The listing builds one solid part. Answer for the finished solid, in the listing's coordinates (mm). A direction names the side the tool comes from. Coordinates: 2 decimals unless noted, no trailing zeros. Write each loop counter-clockwise with the first axis right and the second up, starting at its lowest first coordinate (ties: lowest second). Pieces come first, ordered by that corner, then holes.
Autodesk Inventor part; units mm, degrees
ref_plane "YZ Plane" through (0, 0, 0) normal (1, 0, 0) x (0, 1, 0)
ref_plane "XZ Plane" through (0, 0, 0) normal (0, 1, 0) x (-1, 0, 0)
ref_plane "XY Plane" through (0, 0, 0) normal (0, 0, 1) x (1, 0, 0)
sketch "Sketch1" plane through (0, 0, 0) normal (0, 0, 1) x (1, 0, 0)
  line L0 (-31.75, 5.08) -> (31.75, 5.08)
  line L1 (31.75, 5.08) -> (31.75, -5.08)
  line L2 (31.75, -5.08) -> (-31.75, -5.08)
  line L3 (-31.75, -5.08) -> (-31.75, 5.08)
  point P0 (0, 0)
  dimension "d0" = 63.5
  dimension "d3" = 31.75
  dimension "d4" = 10.16
  dimension "d17" = 5.08
extrude "Extrusion1" add sketch "Sketch1" along normal blind 76.2
sketch "Sketch3" plane through (0, 0, 76.2) normal (0, 0, 1) x (1, 0, 0)
  line L0 (-27.25, 0.3875) -> (27.25, 0.3875)
  line L1 (27.25, 0.3875) -> (27.25, -0.3745)
  line L2 (27.25, -0.3745) -> (-27.25, -0.3745)
  line L3 (-27.25, -0.3745) -> (-27.25, 0.3875)
  line L4 (-31.75, 5.08) -> (-31.75, -5.08)
  point P0 (0, 0)
  point P1 (-27.25, 0.0065)
  dimension "d6" = 0.762
  dimension "d7" = 54.5
  dimension "d8" = 4.5
extrude "Extrusion2" cut sketch "Sketch3" against normal blind 85.1
sketch "Sketch8" plane through (0, 0, 76.2) normal (0, 0, 1) x (1, 0, 0)
  line L0 (-31.75, -5.08) -> (31.75, -5.08)
  line L1 (31.75, -5.08) -> (31.75, 5.08)
  line L2 (-31.75, -5.08) -> (31.75, -5.08)
  line L3 (31.75, -5.08) -> (31.75, 0.3875)
  line L4 (31.75, 0.3875) -> (-31.75, 0.3875)
  line L5 (27.25, 0.3875) -> (27.25, -0.3745)
  line L6 (27.25, -0.3745) -> (-27.25, -0.3745)
  line L7 (-27.25, -0.3745) -> (-27.25, 0.3875)
  line L8 (-27.25, 0.3875) -> (27.25, 0.3875)
  line L9 (-31.75, -5.08) -> (31.75, -5.08)
  line L10 (31.75, -5.08) -> (31.75, 5.08)
  line L11 (31.75, 5.08) -> (-31.75, 5.08)
  line L12 (-31.75, 5.08) -> (-31.75, -5.08)
  line L13 (-27.25, 0.3875) -> (-27.25, -0.3745)
  line L14 (-27.25, 0.3875) -> (27.25, 0.3875)
  line L15 (27.25, 0.3875) -> (27.25, -5.08)
  line L16 (27.25, -5.08) -> (-27.25, -5.08)
  line L17 (-27.25, -5.08) -> (-27.25, 0.3875)
  point P0 (0, 0)
  dimension "d30" = 0
sketch "Sketch9" plane through (-31.75, 5.08, 0) normal (0, 1, 0) x (1, 0, 0)
  line L0 (28.35, -18.7333) -> (35.15, -18.7333)
  line L1 (35.15, -18.7333) -> (35.15, -39.7333)
  line L2 (35.15, -39.7333) -> (28.35, -39.7333)
  line L3 (28.35, -39.7333) -> (28.35, -18.7333)
  line L4 (0, 0) -> (0, -76.2)
  line L5 (63.5, 0) -> (0, 0)
  point P0 (31.75, 0)
  point P1 (0, -38.1)
  dimension "d31" = 21
  dimension "d32" = 6.8
  dimension "d33" = 28.35
  dimension "d34" = 18.7333
extrude "Extrusion6" cut sketch "Sketch8" against normal blind 76.2 contours L17 L6 L15 L0
sketch "Sketch11" plane through (0, 0, 76.2) normal (0, 0, 1) x (1, 0, 0)
  point P0 (0, 0)
sketch "Sketch12" plane through (-31.75, -5.08, 0) normal (0, -1, 0) x (1, 0, 0)
  line L0 (4.5, 0) -> (4.5, 76.2)
  line L1 (0, 76.2) -> (4.5, 76.2)
  line L2 (0, 0) -> (0, 76.2)
  line L3 (0, 0) -> (4.5, 0)
  line L4 (59, 76.2) -> (59, 0)
  line L5 (59, 0) -> (63.5, 0)
  line L6 (63.5, 0) -> (63.5, 76.2)
  line L7 (59, 76.2) -> (63.5, 76.2)
  point P0 (31.75, 0)
extrude "Extrusion7" add sketch "Sketch12" along normal blind 3.641
sketch "Sketch14" plane through (27.25, 0.3875, 0) normal (-1, 0, 0) x (0, 0, 1)
  circle A0 centre (10.16, -3.3935) radius 2.55
  line L0 (76.2, 0) -> (0, 0)
  line L1 (76.2, -9.1085) -> (0, -9.1085)
  line L2 (0, -9.1085) -> (0, 0)
  point P0 (0, -0.3875)
  dimension "d41" = 5.1
  dimension "d43" = 5.715
  dimension "d44" = 10.16
extrude "Extrusion9" cut sketch "Sketch14" against normal blind 25.4
sketch "Sketch17" plane through (-31.75, -8.721, 0) normal (0, -1, 0) x (1, 0, 0)
  circle A0 centre (61.25, 3.81) radius 1.05
  line L0 (59, 0) -> (63.5, 0)
  line L1 (59, 76.2) -> (59, 0)
  circle A1 centre (2.25, 3.81) radius 1.05
  line L2 (0, 76.2) -> (0, 0)
  line L3 (0, 0) -> (4.5, 0)
  circle A2 centre (2.25, 72.39) radius 1.05
  circle A3 centre (61.25, 72.39) radius 1.05
  line L4 (4.5, 76.2) -> (0, 76.2)
  line L5 (63.5, 76.2) -> (59, 76.2)
  point P0 (31.75, 0)
  dimension "d98" = 2.1
  dimension "d99" = 3.81
  dimension "d100" = 2.25
  dimension "d101" = 2.25
  dimension "d102" = 2.1
  dimension "d103" = 3.81
  dimension "d104" = 2.1
  dimension "d105" = 2.1
  dimension "d106" = 3.81
  dimension "d107" = 3.81
  dimension "d108" = 2.25
extrude "Extrusion11" cut sketch "Sketch17" against normal blind 5.08
sketch "Sketch18" plane through (-27.25, 0.3875, 76.2) normal (0, -1, 0) x (1, 0, 0)
  circle A0 centre (5.5, -23.82) radius 1.25
  circle A1 centre (5.5, -12.42) radius 1.05
  circle A2 centre (5.5, -12.42) radius 1.25
  line L0 (3.5, -28.62) -> (3.5, -7.62)
  circle A3 centre (5.5, -23.82) radius 1.05
  line L1 (54.5, -28.62) -> (3.5, -28.62)
  line L2 (3.5, -7.62) -> (54.5, -7.62)
  circle A4 centre (52.5, -12.42) radius 1.05
  circle A5 centre (52.5, -12.42) radius 1.25
  line L3 (54.5, -7.62) -> (54.5, -28.62)
  circle A6 centre (52.5, -23.82) radius 1.05
  circle A7 centre (52.5, -23.82) radius 1.25
  line L4 (0, 0) -> (54.5, 0)
  line L5 (54.5, 0) -> (54.5, -76.2)
  point P0 (27.25, -76.2)
  dimension "d111" = 21
  dimension "d112" = 51
  dimension "d113" = 2.1
  dimension "d114" = 2.1
  dimension "d115" = 2.1
  dimension "d116" = 2.1
  dimension "d117" = 2
  dimension "d118" = 2
  dimension "d119" = 2
  dimension "d120" = 2
  dimension "d121" = 11.4
  dimension "d122" = 4.8
  dimension "d123" = 11.4
  dimension "d124" = 4.8
  dimension "d125" = 0.2
  dimension "d126" = 0.2
  dimension "d127" = 0.2
  dimension "d128" = 0.2
  dimension "d131" = 7.62
  dimension "d132" = 0
extrude "Extrusion12" cut sketch "Sketch18" against normal blind 25.4 contours A0 | A1 | A2 | A3 | A4 | A5 | A6 | A7
sketch "Sketch21" plane through (-31.75, -8.721, 0) normal (0, -1, 0) x (1, 0, 0)
  line L0 (59, 76.2) -> (59, 0)
  line L1 (59, 69.5452) -> (61.2521, 69.5452)
  line L2 (61.2521, 69.5452) -> (61.2521, 46.6852)
  line L3 (61.2521, 46.6852) -> (59, 46.6852)
  line L4 (59, 46.6852) -> (59, 69.5452)
  line L5 (63.5, 0) -> (63.5, 76.2)
  line L6 (63.5, 76.2) -> (59, 76.2)
  point P0 (31.75, 0)
  dimension "d147" = 4.5
  dimension "d148" = 2.2479
  dimension "d149" = 6.6548
  dimension "d150" = 22.86
sketch "Sketch22" plane through (31.75, 5.08, 76.2) normal (1, 0, 0) x (0, 0, -1)
  line L0 (13.67, -4.6925) -> (13.67, 0)
  line L1 (13.67, -4.6925) -> (13.67, 0)
  line L2 (25.07, -4.6925) -> (25.07, 0)
  line L3 (22.57, -4.6925) -> (22.57, 0)
  line L4 (11.17, -4.6925) -> (11.17, 0)
  line L5 (23.8, -2.1525) -> (12.44, -2.1525)
  line L6 (12.44, -2.1525) -> (12.44, -11.0425)
  line L7 (12.44, -11.0425) -> (23.8, -11.0425)
  line L8 (23.8, -11.0425) -> (23.8, -2.1525)
  point P0 (76.2, -5.08)
  point P1 (24.97, -4.6925)
  point P2 (24.97, -2.1525)
  point P3 (11.27, -2.6605)
  point P4 (11.27, -4.6925)
  dimension "d152" = 8.89
  dimension "d153" = 2.54
  dimension "d169" = 1.27
  dimension "d170" = 1.27
extrude "Extrusion15" cut sketch "Sketch22" against normal blind 4.5212
sketch "Sketch24" plane through (31.75, 5.08, 76.2) normal (1, 0, 0) x (0, 0, -1)
  line L0 (38.6849, -4.6925) -> (33.6849, -4.6925)
  line L1 (33.6849, -4.6925) -> (33.6849, -8.6925)
  line L2 (33.6849, -8.6925) -> (38.6849, -8.6925)
  line L3 (38.6849, -8.6925) -> (38.6849, -4.6925)
  line L4 (0, -4.6925) -> (76.2, -4.6925)
  point P0 (76.2, -5.08)
  point P1 (23.8, -4.6925)
  dimension "d163" = 5
  dimension "d164" = 4
  dimension "d165" = 0
extrude "Extrusion16" cut sketch "Sketch24" against normal blind 9.1211
sketch "Sketch27" plane through (-27.25, 0.3875, 76.2) normal (0, -1, 0) x (1, 0, 0)
  line L0 (54.5, 0) -> (54.5, -76.2)
  line L1 (0, 0) -> (0, -76.2)
  line L2 (54.5, -29.89) -> (0, -29.89)
  line L3 (0, -29.89) -> (0, -6.35)
  line L4 (0, -6.35) -> (54.5, -6.35)
  line L5 (54.5, -6.35) -> (54.5, -29.89)
  line L6 (54.5, -28.62) -> (3.5, -28.62)
  line L7 (3.5, -7.62) -> (54.5, -7.62)
  point P0 (27.25, -76.2)
  point P1 (54.5, -6.35)
  point P2 (0, -29.89)
  dimension "d171" = 1.27
  dimension "d172" = 1.27
extrude "Extrusion17" cut sketch "Sketch27" against normal blind 1.5
sketch "Sketch30" plane through (-27.25, 0.3875, 0) normal (0, -1, 0) x (1, 0, 0)
  line L0 (39.9458, 42.5) -> (14.5458, 42.5)
  line L1 (14.5458, 42.5) -> (14.5458, 10.75)
  line L2 (14.5458, 10.75) -> (39.9458, 10.75)
  line L3 (39.9458, 10.75) -> (39.9458, 42.5)
  line L4 (23.85, 39.7333) -> (30.65, 39.7333)
  line L5 (54.5, 0) -> (0, 0)
  line L6 (54.5, 76.2) -> (54.5, 0)
  line L7 (0, 0) -> (0, 76.2)
  line L8 (36.9458, 38) -> (17.5458, 38)
  line L9 (17.5458, 38) -> (17.5458, 15.25)
  line L10 (17.5458, 15.25) -> (36.9458, 15.25)
  line L11 (36.9458, 15.25) -> (36.9458, 38)
  circle A0 centre (37.9458, 40.5) radius 1.25
  line L12 (54.5, 46.31) -> (0, 46.31)
  circle A1 centre (37.9458, 12.75) radius 1.25
  circle A2 centre (16.5458, 12.75) radius 1.25
  circle A3 centre (16.5458, 40.5) radius 1.25
  line L13 (54.5, 46.31) -> (0, 46.31)
  line L14 (0, 46.31) -> (0, 0)
  line L15 (54.5, 0) -> (0, 0)
  line L16 (54.5, 37.5151) -> (54.5, 0)
  line L17 (59, 37.5151) -> (54.5, 37.5151)
  line L18 (59, 42.5151) -> (59, 37.5151)
  line L19 (59, 42.5151) -> (54.5, 42.5151)
  line L20 (54.5, 46.31) -> (54.5, 42.5151)
  line L21 (41.8508, 44.405) -> (12.6408, 44.405)
  line L22 (12.6408, 44.405) -> (12.6408, 8.845)
  line L23 (12.6408, 8.845) -> (41.8508, 8.845)
  line L24 (41.8508, 8.845) -> (41.8508, 44.405)
  point P0 (27.25, 0)
  dimension "d177" = 31.75
  dimension "d178" = 25.4
  dimension "d179" = 54.5
  dimension "d180" = 14.5542
  dimension "d181" = 4.5
  dimension "d182" = 3.81
  dimension "d183" = 3
  dimension "d184" = 4.5
  dimension "d185" = 3
  dimension "d186" = 2.5
  dimension "d187" = 2
  dimension "d188" = 2
  dimension "d189" = 2.5
  dimension "d190" = 2.5
  dimension "d191" = 2.5
  dimension "d193" = 2
  dimension "d195" = 2
  dimension "d196" = 2
  dimension "d197" = 2
  dimension "d204" = 1.905
  dimension "d210" = 2
  dimension "d211" = 2
extrude "Extrusion18" cut sketch "Sketch30" against normal blind 25.4 contours L11 L10 L9 L8
extrude "Extrusion19" cut sketch "Sketch30" against normal blind 1.5 contours L3 L2 L1 L0 | L11 L10 L9 L8 | A0 | A1 | A2 | A3 | L24 L23 L22 L21
extrude "Extrusion20" cut sketch "Sketch30" against normal blind 254 contours A0 | A1 | A2 | A3
properties part number "Scanner_Test_Top"
1. Find the intervals of material crossed by L1, parallel to Z at x = -29.5, y = -6.8; L2, parallel to X at y = -6, z = 34.5; L3, parallel to Z at x = -5.5, y = 3, in increasing order.
Results found:
L1: z = 0 to 2.76, 4.86 to 71.34, 73.44 to 76.2
L2: x = -31.75 to -27.25, 27.25 to 31.75
L3: z = 0 to 15.25, 38 to 76.2
2. Section A-A on x = 25.25 is taken. Give the vertices of the cut face in (y, z).
Results found:
outline: (0.39, 0) - (5.08, 0) - (5.08, 51.13) - (1.89, 51.13) - (1.89, 46.31) - (0.39, 46.31) - close; (0.39, 69.85) - (1.89, 69.85) - (1.89, 65.03) - (5.08, 65.03) - (5.08, 76.2) - (0.39, 76.2) - close; (1.89, 53.63) - (5.08, 53.63) - (5.08, 62.53) - (1.89, 62.53) - close
3. Flat-ended cylindrical pins translate along their axes: P1, Ø4, axis at x = -21.75, z = 63.78, coming from the -Y side; P2, Ø8, axis at x = -15, z = 12, coming from the -Y side; P3, Ø0.6, axis at x = -29.5, z = 73, coming from the -Y side; P4, Ø2, axis at x = 25.25, z = 52.38, coming from the -Y side. Find the tip coordinate at first contact, or state that the pin passes through.
Results found:
P1: stops at y = 1.89
P2: stops at y = 0.39
P3: stops at y = -3.64
P4: passes through
4. Section D-D on y = -1.5 is taken. Give the vertices of the cut face in (x, z).
Results found:
outline: (-31.75, 0) - (-27.25, 0) - (-27.25, 76.2) - (-31.75, 76.2) - close; (27.25, 0) - (31.75, 0) - (31.75, 8.1) - (27.25, 8.1) - close; (27.25, 12.22) - (31.75, 12.22) - (31.75, 37.52) - (27.25, 37.52) - close; (27.25, 42.52) - (31.75, 42.52) - (31.75, 52.4) - (27.25, 52.4) - close; (27.25, 63.76) - (31.75, 63.76) - (31.75, 76.2) - (27.25, 76.2) - close
5. A tool of negligible diameter and unlimited length cuts with its end or side. For faces 5 (the flat face through (0, 0.388, 73)), 6 (the flat face through (0, 3, 15.25)), 7 (the flat face through (31.75, -5, 38)), 8 (the cylindrical face through (30.5, -6.22, 4.13)), 9 (the flat face through (30, -5.962, 58)), from which of +Z, -Z, +X, -X, +Y, -Y can it reach the whole face along a straight path? Write none if from no direction.
Results found:
face 5: +Z, -Z, -Y
face 6: +Y, -Y
face 7: +Z, -Z, +X, +Y, -Y
face 8: -Y
face 9: +X
6. Section B-B on z = 10.16 is taken. Give the vertices of the cut face in (x, y), then the cut area to 3 significant figures.
Results found:
outline: (-31.75, -8.72) - (-27.25, -8.72) - (-27.25, 0.39) - (-14.61, 0.39) - (-14.61, 1.89) - (14.6, 1.89) - (14.6, 0.39) - (27.25, 0.39) - (27.25, -0.46) - (31.75, -0.46) - (31.75, 5.08) - (-31.75, 5.08) - close; (27.25, -8.72) - (31.75, -8.72) - (31.75, -5.56) - (27.25, -5.56) - close
area: 313 mm2
7. For a pull along Z with two mould halves and no side action, classify faces 1 (the flat face through (0, 5.08, 46)), 2 (the flat face through (0, 1, 0)), 3 (the cylindrical face through (-20.595, 3.461, 63.301)), 4 (the cylindrical face through (9.77, 3.46, 13.59)) as pulls with the +Z half, pulls with the -Z half, needs draft (parallel to the pull), parting line crosses it, or undercut.
Results found:
face 1: needs draft
face 2: pulls with the -Z half
face 3: undercut
face 4: undercut
